from build123d import *

# Parameters (mm, degrees)
F1_DEPTH = 65
F2_R     = 7.5
F3_DEPTH = 25
F5_DEPTH = 15.5081460252
F8_DEPTH = 4.1
F9_R     = 5


with BuildPart() as f1:
    # F0 (on Right) → F1 (new body)
    with BuildSketch(Plane.YZ):
        Polygon((-64.9103820324, 0), (0, 0), (0, 67.3085525632), (-21.7433813959, 67.3085525632), (-21.7433813959, 15.5081460252), (-64.9103820324, 15.5081460252), align=None)
    extrude(amount=F1_DEPTH)

    # F2 (on face) → F3 (cut)
    with BuildSketch(Plane.XZ.offset(21.7433813959)):
        with Locations((32.5, 54.9736991525)):
            Circle(F2_R)
    extrude(amount=-F3_DEPTH, mode=Mode.SUBTRACT)

    # F4 (on face) → F5 (cut, through all)
    with BuildSketch(Plane.XY.offset(15.5081460252)):
        with BuildLine():
            Line((42.4322629764, -64.9103820324), (42.4322629764, -46.9211071186))
            ThreePointArc((42.4322629764, -46.9211071186), (32.5, -35.7591466337), (22.5677370236, -46.9211071186))
            Line((22.5677370236, -46.9211071186), (22.5677370236, -64.9103820324))
            Line((22.5677370236, -64.9103820324), (42.4322629764, -64.9103820324))
        make_face()
    extrude(amount=-F5_DEPTH, mode=Mode.SUBTRACT)

    # F7 (on offset) → F8 (join, symmetric)
    with BuildSketch(Plane.YZ.offset(55)):
        Polygon((-21.7433813959, 15.5081460252), (-21.7433813959, 47.5081460252), (-33.7433813959, 15.5081460252), align=None)
    extrude(amount=F8_DEPTH, both=True)

    # F9
    f9_edges = [f1.edges().sort_by_distance(p)[0] for p in [
        (0, -10.871691, 67.308553),
        (65, -10.871691, 67.308553),
        (11.283869, -64.910382, 15.508146),
        (0, -43.326882, 15.508146),
        (0, -21.743381, 41.408349),
        (0, 0, 33.654276),
        (0, -32.455191, 0),
        (11.283869, -64.910382, 0),
        (65, -64.910382, 7.754073),
        (65, -43.326882, 15.508146),
        (65, -21.743381, 41.408349),
        (65, 0, 33.654276),
        (65, -32.455191, 0),
        (42.432263, -64.910382, 7.754073),
        (53.716131, -64.910382, 0),
        (53.716131, -64.910382, 15.508146),
        (55, -33.743381, 15.508146),
    ]]
    fillet(f9_edges, radius=F9_R)


solid = f1.part
Can you work these out from the model? Positions are in its coordinate system, mm. A direction names the side the tool comes from. Give positions to 0.01 mm unless a question says otherwise; leave off trailing zeros. Order: outer loops, then holes, each group sorted by start corner. A loop starts at its lowest first (then second) coordinate and runs counter-clockwise, first axis right, second up. Notation, with made-up numbers: (-26, 78) - (-1, 78) arc R20 cw to (-1, 83) - close; hole circle Ø3 at (74, 31.25). An arc over 180 degrees is marked (long way). Write each question's results on one line, items separated by ' | '.
1) I'm going to push flat-ended pins straight in: pin 1 Ø19 at (x, y) = (24.5, -35) entering from +Z; pin 2 Ø7.5 at (y, z) = (-33.5, 27.5) entering from -X; pin 3 Ø3 at (x, z) = (21, 39) entering from -Y; pin 4 Ø7.5 at (y, z) = (-30, 29) entering from +X. Where does each tip first touch, or does it pass through?
Final values:
pin 1: stops at z = 15.51 | pin 2: passes through | pin 3: stops at y = -21.74 | pin 4: stops at x = 59.1
2) Suppose I cut it at A-A, the plane x = 32.5. Write out the boundary of the cut face in (y, z).
Final values:
outline: (-35.76, 0) - (0, 0) - (0, 47.47) - (-21.74, 47.47) - (-21.74, 15.51) - (-35.76, 15.51) - close; (-21.74, 62.47) - (0, 62.47) - (0, 67.31) - (-21.74, 67.31) - close
3) Suppose I cut it at D-D, the plane z = 42. Write out the boundary of the cut face in (x, y), then the cut area to 3 significant figures.
Final values:
outline: (0, -16.74) arc R5 ccw to (5, -21.74) - (50.9, -21.74) - (50.9, -23.81) - (59.1, -23.81) - (59.1, -21.74) - (60, -21.74) arc R5 ccw to (65, -16.74) - (65, -5) arc R5 ccw to (60, 0) - (5, 0) arc R5 ccw to (0, -5) - close | area: 1,410 mm^2
4) If we mould it in two halves opening along X, with no side actions, what happens to faces 1 (the face through (22.568, -56, 8)), 2 (the face through (51.339, -63.485, 14.005)), 3 (the face through (59.1, -26, 25))? For each: pulls with the +X half, pulls with the -X half, needs draft (parallel to the pull), parting line crosses it, or undercut.
Final values:
face 1: undercut | face 2: needs draft | face 3: pulls with the +X half
5) Suppose I cut it at C-C, the plane x = 57. Write out the boundary of the cut face in (y, z), then the cut area to 3 significant figures.
Final values:
outline: (-64.91, 5) arc R5 ccw to (-59.91, 0) - (0, 0) - (0, 67.31) - (-21.74, 67.31) - (-21.74, 47.51) - (-32.53, 18.75) arc R5 cw to (-37.21, 15.51) - (-59.91, 15.51) arc R5 ccw to (-64.91, 10.51) - close | area: 2,320 mm^2
6) Please list where these lines run through material, in increasing order: line 1 along X through (y, z) = (-60, 9); line 2 along Z through (x, y) = (14.5, -45); line 3 along Y through (x, z) = (20, 45.5). Write a range as [from, to].
Final values:
line 1: x = [0, 22.57], [42.43, 65] | line 2: z = [0, 15.51] | line 3: y = [-21.74, 0]
7) Suppose I cut it at B-B, the plane z = 49. Write out the boundary of the cut face in (x, y).
Final values:
outline: (0, -16.74) arc R5 ccw to (5, -21.74) - (27.97, -21.74) - (27.97, 0) - (5, 0) arc R5 ccw to (0, -5) - close; (37.03, -21.74) - (60, -21.74) arc R5 ccw to (65, -16.74) - (65, -5) arc R5 ccw to (60, 0) - (37.03, 0) - close
8) On a 3-axis mill with a long thin cutter (end or side, diameter ignored), from which of +Z, -Z, +X, -X, +Y, -Y can I reach the whole of each face in a straight line? I mean faces 4 (the face through (1.426, -20.24, 38.511)), 5 (the face through (43.368, -62.823, 7.646)), 6 (the face through (32.736, -35.762, 7.863)). Say none if no direction works.
Final values:
face 4: +Z, -X, -Y | face 5: +Z, -Z, -Y | face 6: +Z, -Z
